Part model, mm, in its own coordinate system. A direction names the side the tool comes from. Round coordinates to 2 decimals unless told otherwise and drop trailing zeros. Loops run counter-clockwise (first coordinate to the right, second up) from the corner with the lowest first, then second, coordinate; pieces in that order, holes last. Notation, with made-up numbers: (71, 44) -> (93, 44) arc R25 ccw to (93, 78) -> close; hole circle Ø6 at (-30.5, 87.25). An arc over 180 degrees is marked (long way). Answer as CSV lines item,"result".
from build123d import *

# Parameters (mm, degrees)
F1_DEPTH = 3.75


# Not quite as in the source:
# - a feature of the source that left no trace in its solid (it failed there, or was rolled back) is left out


with BuildPart() as f1:
    # F0 (on Top) → F1 (new body)
    with BuildSketch(Plane.XY):
        with BuildLine():
            Line((11.2, 144.2591021933), (11.2, 147.0741649645))
            ThreePointArc((11.2, 147.0741649645), (0, 147.5), (-11.2, 147.0741649645))
            Line((-11.2, 147.0741649645), (-11.2, 144.2591021933))
            ThreePointArc((-11.2, 144.2591021933), (-11.3222315822, 143.9291191636), (-11.6299352058, 143.7583917795))
            Line((-11.6299352058, 143.7583917795), (-14.7849675268, 143.2757224802))
            Line((-14.7849675268, 143.2757224802), (-14.7849675268, 142.5268018024))
            Line((-14.7849675268, 142.5268018024), (-11.2, 142.5268018024))
            Line((-11.2, 142.5268018024), (11.2, 142.5268018024))
            Line((11.2, 142.5268018024), (14.7849675268, 142.5268018024))
            Line((14.7849675268, 142.5268018024), (14.7849675268, 143.2757224802))
            Line((14.7849675268, 143.2757224802), (11.6299352058, 143.7583917795))
            ThreePointArc((11.6299352058, 143.7583917795), (11.3222315822, 143.9291191636), (11.2, 144.2591021933))
        make_face()
    extrude(amount=F1_DEPTH)


solid = f1.part
Q1. Saw through at A-A, the plane z = 1.7. Write the cut outline in (x, y).
Geometry results:
outline,"(-14.78, 142.53) -> (14.78, 142.53) -> (14.78, 143.28) -> (11.63, 143.76) arc R0.51 cw to (11.2, 144.26) -> (11.2, 147.07) arc R147.5 ccw to (-11.2, 147.07) -> (-11.2, 144.26) arc R0.51 cw to (-11.63, 143.76) -> (-14.78, 143.28) -> close"
Q2. Drop flat-ended pins along their axis: P1, Ø2, axis at x = 4, z = 3, coming from the +Y side; P2, Ø0.8, axis at y = 146, z = 1, coming from the +X side. Give the stop position or say it passes through.
Geometry results:
P1,"y = 147.47"
P2,"x = 11.2"
Q3. Drill centre lines: line 1 along X through (y, z) = (146.45, 2.75); line 2 along Y through (x, z) = (3.5, 0.95); line 3 along Y through (x, z) = (-10.25, 2.9). Where is each one in solid material? Low to high.
Geometry results:
line 1,"-11.2 to 11.2"
line 2,"142.53 to 147.46"
line 3,"142.53 to 147.14"
Q4. Saw through at B-B, the plane y = 144.8. Write the cut outline in (x, z).
Geometry results:
outline,"(-11.2, 0) -> (11.2, 0) -> (11.2, 3.75) -> (-11.2, 3.75) -> close"
Q5. Which spindle directions (+Z, -Z, +X, -X, +Y, -Y) get a long thin tool onto all of the face, cutting with end or side? Do faces 1 (the face through (0.2, 147.5, 1.8)), 2 (the face through (11.2, 146, 2)), 3 (the face through (-11.2, 146, 2)). Say none if no direction does.
Geometry results:
face 1,"+Z, -Z, +Y"
face 2,"+Z, -Z, +X, +Y"
face 3,"+Z, -Z, -X, +Y"
Q6. Saw through at C-C, the plane x = 8.25. Write the cut outline in (y, z), then the cut area to 3 significant figures.
Geometry results:
outline,"(142.53, 0) -> (147.27, 0) -> (147.27, 3.75) -> (142.53, 3.75) -> close"
area,"17.8 mm2"
